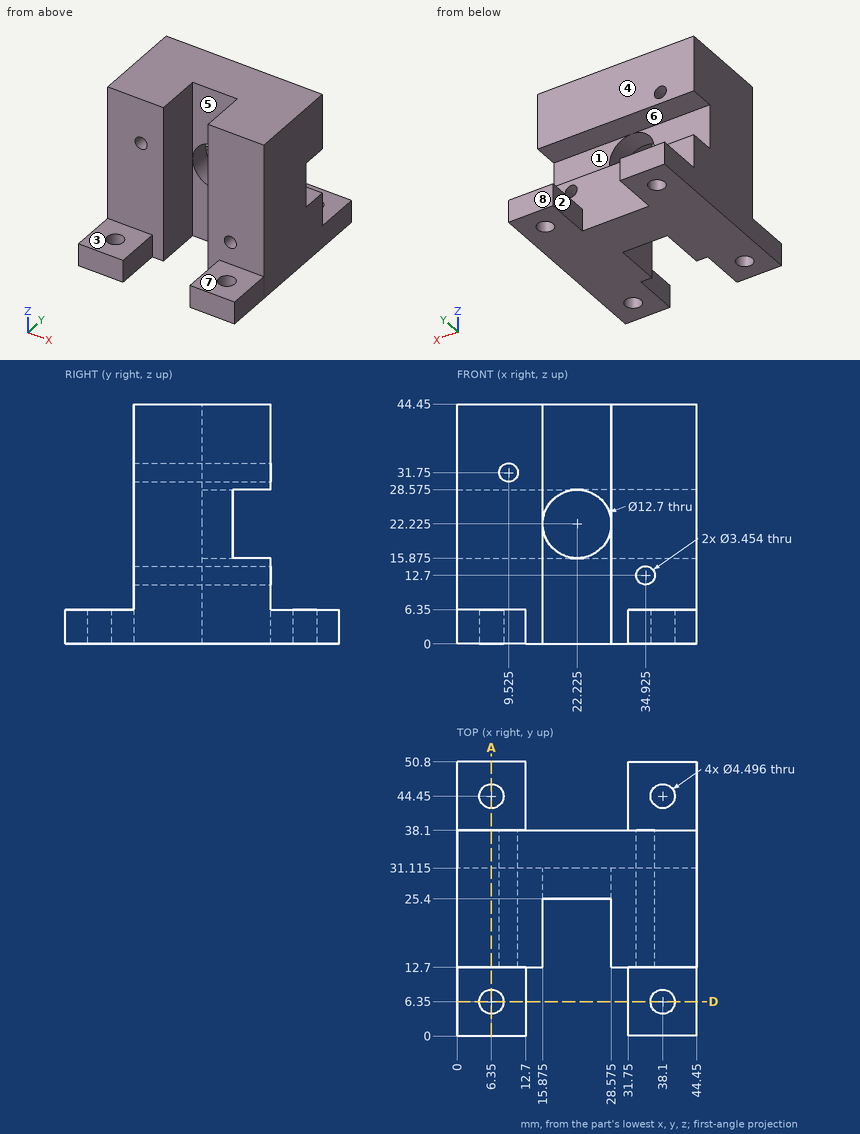
For this review, use the dimensioned drawing (mm, ordinates from the lowest corner) and the shaded views. A direction names the side the tool comes from. Give positions to 0.01 mm unless a question says otherwise; leave off trailing zeros. Order: outer loops, then holes, each group sorted by start corner. A loop starts at its lowest first (then second) coordinate and runs counter-clockwise, first axis right, second up. Notation, with made-up numbers: (61, -15) - (116, -15) arc R27 ccw to (116, 3) - close; hole circle Ø10 at (18.5, 80). An arc over 180 degrees is marked (long way). Use CSV: the item, a comma, the result in double quotes. Start each with the question number.
Q1. We need section A-A, the plane x = 6.35. State how many separate pieces and enclosed holes the cut face has, and give its area (3 significant figures).
Q2. The part is to be moulded in two halves that separate along Z. For the marked faces 6, 7 and 8, say which applies: +Z half, -Z half, draft (parallel to the pull), parting line (faces both ways), or undercut.
Q3. We need section D-D, the plane y = 6.35. Write out the cut boundary in (x, z), and give its area (3 significant figures).
Q4. Tool access review of the marked faces 1, 2, 3, 4 and 5: name each direction out of +Z, -Z, +X, -X, +Y, -Y from which nothing blocks a thin tool from reaching the whole face with its end or side.
Q5. Clearance check with flat-ended pins moving along their axes: pin 1 Ø2 at (y, z) = (11.5, 15.5) entering from +X; pin 2 Ø5 at (x, z) = (32, 36.5) entering from -Y; pin 3 Ø4 at (x, y) = (36.5, 5) entering from +Z; pin 4 Ø6.5 at (x, z) = (28, 20) entering from +Y (3 decimals). State where each tip first meets the part, or that it passes through.
Q6. To check wall thickness, follow line 1 along Y through (x, z) = (38.1, 1.5); line 2 along X through (y, z) = (6, 5); line 3 along Y through (x, z) = (37.5, 3.5). State the ranges of each line that lie inside material, in increasing order. Write a range as [from, to].
Outcome:
1,separate pieces,"3"
1,enclosed holes,"0"
1,area,"1,140 mm^2"
2,face 6,"undercut"
2,face 7,"+Z half"
2,face 8,"draft"
3,outline,"(0, 0) - (4.1, 0) - (4.1, 6.35) - (0, 6.35) - close; (8.6, 0) - (12.7, 0) - (12.7, 6.35) - (8.6, 6.35) - close; (31.75, 0) - (35.85, 0) - (35.85, 6.35) - (31.75, 6.35) - close; (40.35, 0) - (44.45, 0) - (44.45, 6.35) - (40.35, 6.35) - close"
3,area,"104 mm^2"
4,face 1,"+X, -X, +Y"
4,face 2,"+Z, -Z, +Y"
4,face 3,"+Z, +X, -X, -Y"
4,face 4,"+Z, +X, -X, +Y"
4,face 5,"+Z, -Z, -Y"
5,pin 1,"passes through"
5,pin 2,"stops at y = 12.7"
5,pin 3,"stops at z = 6.35"
5,pin 4,"stops at y = 31.115"
6,line 1,"y = [0, 4.1], [8.6, 42.2], [46.7, 50.8]"
6,line 2,"x = [0, 4.13], [8.57, 12.7], [31.75, 35.88], [40.32, 44.45]"
6,line 3,"y = [0, 4.18], [8.52, 42.28], [46.62, 50.8]"
